The listing builds one solid part. Answer for the finished solid, in the listing's coordinates (mm). A direction names the side the tool comes from. Round coordinates to 2 decimals unless told otherwise and drop trailing zeros. Order: outer loops, then holes, each group sorted by start corner. A loop starts at its lowest first (then second) coordinate and runs counter-clockwise, first axis right, second up. Notation, with made-up numbers: M 87,67.5 L 128,67.5 A25 cw 128,96.5 Z; hole C -34,12.25 d6. An arc over 180 degrees is marked long. Write item = value, one per line. Start each with the question number.
(1) For a pull along Z with two mould halves and no side action, classify faces 1 (the face through (-84.26, 3.13, 0.73)), 2 (the face through (-68, 3, 17.249)), 3 (the face through (-163.17, 3, 3)) as released by +Z, released by -Z, zero draft, split by the parting line, or undercut.
(2) Which of the six approach directions +Z, -Z, +X, -X, +Y, -Y give full straight-line access (tool end or side, diameter ignored) to faces 4 (the face through (-109, 6.35, 12)), 5 (the face through (-166, 3, -1.166)), 6 (the face through (-134.637, 3, 23)), 7 (the face through (-169.52, 3, -4)), 8 (the face through (-64.622, 3, 20))?
(3) A cutting plane is placed at A-A, the plane x = -103. Determine the outline of the cut face in (y, z), and give its area (3 significant figures).
(4) Straight lines are drawn through the part: probe 1 along Z at (x, y) = (-161, 2.5); probe 2 along X at (y, z) = (3, 21); probe 3 along X at (y, z) = (1.25, 22). For each, find the intervals that lie inside material, in ascending order. Write a range as from..to.
(5) Each of these flat-tipped pins is pushed along its axis until it touches: pin 1 (1.4 mm diameter, centred on x = -138.5, y = 4.5, fed in from -Z); pin 2 (0.5 mm diameter, centred on x = -134, y = 4, fed in from -Z); pin 3 (2 mm diameter, centred on y = 2.5, z = 2.5, fed in from -X). Where does it stop, or does it pass through?
(6) A cutting plane is placed at B-B, the plane z = 1.5. Determine the outline of the cut face in (x, y), and give its area (3 significant figures).
from build123d import *

# Parameters (mm, degrees)
BOSS_EXTRUDE1_DEPTH = 6.35


with BuildPart() as part:
    # Sketch1 → Boss-Extrude1 (new body)
    with BuildSketch(Plane(origin=(0, 0, 0), x_dir=(1, 0, 0), z_dir=(0, 1, 0))):
        with BuildLine():
            Line((-163.169535376, 1.165732309), (-163.169535376, -6.882681502))
            Line((-163.169535376, -6.882681502), (-159.994535376, -6.882681502))
            Line((-159.994535376, -6.882681502), (-159.994535376, -5.130081502))
            Line((-159.994535376, -5.130081502), (-157.454535376, -5.130081502))
            Line((-157.454535376, -5.130081502), (-157.454535376, -6.882681502))
            Line((-157.454535376, -6.882681502), (-156.184535376, -6.882681502))
            Line((-156.184535376, -6.882681502), (-156.184535376, -9.930540858))
            Line((-156.184535376, -9.930540858), (-157.454535376, -9.930540858))
            Line((-157.454535376, -9.930540858), (-157.454535376, -11.683140858))
            Line((-157.454535376, -11.683140858), (-159.994535376, -11.683140858))
            Line((-159.994535376, -11.683140858), (-159.994535376, -9.930540858))
            Line((-159.994535376, -9.930540858), (-163.169535376, -9.930540858))
            Line((-163.169535376, -9.930540858), (-163.169535376, -17.884267691))
            Line((-163.169535376, -17.884267691), (-169.519535376, -17.884267691))
            Line((-169.519535376, -17.884267691), (-169.519535376, -24.234267691))
            Line((-169.519535376, -24.234267691), (-137.68483349, -24.234267691))
            Line((-137.68483349, -24.234267691), (-137.68483349, -21.059267691))
            Line((-137.68483349, -21.059267691), (-139.43743349, -21.059267691))
            Line((-139.43743349, -21.059267691), (-139.43743349, -18.519267691))
            Line((-139.43743349, -18.519267691), (-137.68483349, -18.519267691))
            Line((-137.68483349, -18.519267691), (-137.68483349, -17.249267691))
            Line((-137.68483349, -17.249267691), (-134.636974134, -17.249267691))
            Line((-134.636974134, -17.249267691), (-134.636974134, -18.519267691))
            Line((-134.636974134, -18.519267691), (-132.884374134, -18.519267691))
            Line((-132.884374134, -18.519267691), (-132.884374134, -21.059267691))
            Line((-132.884374134, -21.059267691), (-134.636974134, -21.059267691))
            Line((-134.636974134, -21.059267691), (-134.636974134, -24.234267691))
            Line((-134.636974134, -24.234267691), (-69.42233349, -24.234267691))
            Line((-69.42233349, -24.234267691), (-69.42233349, -21.059267691))
            Line((-69.42233349, -21.059267691), (-71.17493349, -21.059267691))
            Line((-71.17493349, -21.059267691), (-71.17493349, -18.519267691))
            Line((-71.17493349, -18.519267691), (-69.42233349, -18.519267691))
            Line((-69.42233349, -18.519267691), (-69.42233349, -17.249267691))
            Line((-69.42233349, -17.249267691), (-66.374474134, -17.249267691))
            Line((-66.374474134, -17.249267691), (-66.374474134, -18.519267691))
            Line((-66.374474134, -18.519267691), (-64.621874134, -18.519267691))
            Line((-64.621874134, -18.519267691), (-64.621874134, -21.059267691))
            Line((-64.621874134, -21.059267691), (-66.374474134, -21.059267691))
            Line((-66.374474134, -21.059267691), (-66.374474134, -24.234267691))
            Line((-66.374474134, -24.234267691), (-10.769535376, -24.234267691))
            ThreePointArc((-10.769535376, -24.234267691), (-85.333453608, -0.506075205), (-163.169535376, 7.515732309))
            Line((-163.169535376, 7.515732309), (-169.519535376, 7.515732309))
            Line((-169.519535376, 7.515732309), (-169.519535376, 1.165732309))
            Line((-169.519535376, 1.165732309), (-163.169535376, 1.165732309))
        make_face()
    extrude(amount=BOSS_EXTRUDE1_DEPTH)


solid = part.part
Reported:
q1.face_1 = released by -Z
q1.face_2 = released by +Z
q1.face_3 = undercut
q2.face_4 = +Z, -Z, +X, -X, +Y
q2.face_5 = -X, +Y, -Y
q2.face_6 = +Z, +Y, -Y
q2.face_7 = +Z, -Z, -X, +Y, -Y
q2.face_8 = +Y, -Y
q3.outline = M 0,-2.74 L 6.35,-2.74 L 6.35,24.23 L 0,24.23 Z
q3.area = 171 mm²
q4.probe_1 = -7.51..6.88, 9.93..24.23
q4.probe_2 = -169.52..-139.44, -132.88..-71.17, -64.62..-18.42
q4.probe_3 = -169.52..-137.68, -134.64..-69.42, -66.37..-16.01
q5.pin_1 = -6.76
q5.pin_2 = -6.42
q5.pin_3 = -163.17
q6.outline = M -163.17,0 L -80.71,0 L -80.71,6.35 L -163.17,6.35 Z
q6.area = 524 mm²
